from build123d import *

# Parameters (mm, degrees)
BOSS_EXTRUDE1_DEPTH     = 25.4
SKETCH2_W               = 12.7
SKETCH2_H               = 12.7
CUT_EXTRUDE1_DEPTH      = 12.7
MIRROR2_COPY_1_SKETCH_W = 12.7
MIRROR2_COPY_1_SKETCH_H = 12.7
MIRROR2_COPY_1_DEPTH    = 12.7
SKETCH3_R               = 3.175
CUT_EXTRUDE2_DEPTH      = 51.252303648


with BuildPart() as part:
    # Sketch1 → Boss-Extrude1 (new body)
    with BuildSketch(Plane.XY):
        Polygon((-30.660512242, 12.7), (-30.660512242, -12.7), (-12.7, -30.660512242), (12.7, -30.660512242), (30.660512242, -12.7), (30.660512242, 12.7), (12.7, 30.660512242), (-12.7, 30.660512242), align=None)
    extrude(amount=BOSS_EXTRUDE1_DEPTH)

    # Sketch2 → Cut-Extrude1 (cut)
    with BuildSketch(Plane(origin=(21.680256121, 21.680256121, 0), x_dir=(0, 0, -1), z_dir=(0.7071067811865479, 0.7071067811865472, 0))):
        with Locations((-12.7, 0)):
            Rectangle(SKETCH2_W, SKETCH2_H)
    cut_extrude1 = extrude(amount=-CUT_EXTRUDE1_DEPTH, mode=Mode.SUBTRACT)

    # Mirror1: Cut-Extrude1 across plane
    add(cut_extrude1.mirror(Plane(origin=(0, 0, 0), x_dir=(0, 0, 1), z_dir=(1, 0, 0))), mode=Mode.SUBTRACT)

    # Mirror2: Cut-Extrude1 across plane
    add(cut_extrude1.mirror(Plane.ZX), mode=Mode.SUBTRACT)

    # Mirror2 copy 1 sketch → Mirror2 copy 1 (cut)
    with BuildSketch(Plane(origin=(-21.680256121, -21.680256121, 0), x_dir=(0, 0, -1), z_dir=(-0.7071067811865472, -0.7071067811865479, 0))):
        with Locations((-12.7, 0)):
            Rectangle(MIRROR2_COPY_1_SKETCH_W, MIRROR2_COPY_1_SKETCH_H)
    extrude(amount=-MIRROR2_COPY_1_DEPTH, mode=Mode.SUBTRACT)

    # Sketch3 → Cut-Extrude2 (cut, through all)
    with BuildSketch(Plane.XY.offset(25.4)):
        with Locations((-17.190128061, 17.190128061)):
            Circle(SKETCH3_R)
        with Locations(Location((-17.190128061, -17.190128061, 0), (0, 0, 180))):
            Circle(SKETCH3_R)
        with Locations((17.190128061, -17.190128061)):
            Circle(SKETCH3_R)
        with Locations(Location((17.190128061, 17.190128061, 0), (0, 0, 180))):
            Circle(SKETCH3_R)
    extrude(amount=-CUT_EXTRUDE2_DEPTH, mode=Mode.SUBTRACT)


solid = part.part
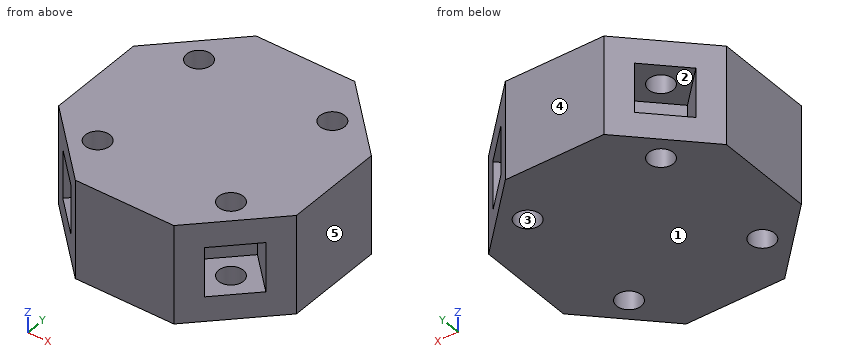
The listing builds one solid part. Answer for the finished solid, in the listing's coordinates (mm). Face numbers are marked on the shaded views. A direction names the side the tool comes from. Coordinates: 2 decimals unless noted, no trailing zeros. Loops run counter-clockwise (first coordinate to the right, second up) from the corner with the lowest first, then second, coordinate; pieces in that order, holes last.
1) Determine the mould class of the marked faces 3, 4 and 5 for opening direction X: pulls with the +X half, pulls with the -X half, needs draft (parallel to the pull), parting line crosses it, or undercut.
2) Find section D-D on x = 10. Write down the section's boundary in (y, z).
3) Find the intervals of material crossed by L1, parallel to Y at x = -17, z = 11; L2, parallel to Y at x = 9, z = 11; L3, parallel to X at y = -15.5, z = 1.25, in increasing order.
4) A tool of negligible diameter and unlimited length cuts with its end or side. For the marked faces 1 and 2, from which of +Z, -Z, +X, -X, +Y, -Y can it reach the whole face along a straight path? Write none if from no direction.
5) Find section B-B on x = -16. Write down the section's boundary in (y, z), then the cut area to 3 significant figures.
6) Flat-ended cylindrical pins translate along their axes: pin 1 Ø8 at (x, z) = (-24, 20.5) entering from +Y; pin 2 Ø9 at (x, y) = (15.5, -16.5) entering from -Z; pin 3 Ø4 at (x, z) = (-24, 17.5) entering from -Y; pin 4 Ø1 at (y, z) = (-21.5, 21.5) entering from +X. Find the tip coordinate at first contact, or state that the pin passes through.
7) Find section C-C on z = 13. Write down the section's boundary in (x, y), then the cut area to 3 significant figures.
8) Find section A-A on z = 22.25. Write down the section's boundary in (x, y) (3 decimals).
Values:
1. face 3: undercut
1. face 4: needs draft
1. face 5: pulls with the +X half
2. outline: (-30.66, 0) - (30.66, 0) - (30.66, 25.4) - (-30.66, 25.4) - close; hole (-18.98, 6.35) - (-15.4, 6.35) - (-15.4, 19.05) - (-18.98, 19.05) - close; hole (15.4, 6.35) - (18.98, 6.35) - (18.98, 19.05) - (15.4, 19.05) - close
3. L1: y = -26.36 to -25.98, -8.4 to 8.4, 25.98 to 26.36
3. L2: y = -30.66 to -17.98, -16.4 to 16.4, 17.98 to 30.66
3. L3: x = -27.86 to -19.88, -14.5 to 14.5, 19.88 to 27.86
4. face 1: -Z, +X, -X, +Y, -Y
4. face 2: none
5. outline: (-27.36, 0) - (-20.13, 0) - (-20.13, 6.35) - (-24.98, 6.35) - (-24.98, 19.05) - (-20.13, 19.05) - (-20.13, 25.4) - (-27.36, 25.4) - close; (-14.25, 0) - (14.25, 0) - (14.25, 6.35) - (9.4, 6.35) - (9.4, 19.05) - (14.25, 19.05) - (14.25, 25.4) - (-14.25, 25.4) - (-14.25, 19.05) - (-9.4, 19.05) - (-9.4, 6.35) - (-14.25, 6.35) - close; (20.13, 0) - (27.36, 0) - (27.36, 25.4) - (20.13, 25.4) - (20.13, 19.05) - (24.98, 19.05) - (24.98, 6.35) - (20.13, 6.35) - close
5. area: 845 mm2
6. pin 1: stops at y = 23.36
6. pin 2: stops at z = 0
6. pin 3: stops at y = -20.62
6. pin 4: stops at x = 22.36
7. outline: (-30.66, -12.7) - (-26.17, -17.19) - (-17.19, -8.21) - (-8.21, -17.19) - (-17.19, -26.17) - (-12.7, -30.66) - (12.7, -30.66) - (17.19, -26.17) - (8.21, -17.19) - (17.19, -8.21) - (26.17, -17.19) - (30.66, -12.7) - (30.66, 12.7) - (26.17, 17.19) - (17.19, 8.21) - (8.21, 17.19) - (17.19, 26.17) - (12.7, 30.66) - (-12.7, 30.66) - (-17.19, 26.17) - (-8.21, 17.19) - (-17.19, 8.21) - (-26.17, 17.19) - (-30.66, 12.7) - close
7. area: 2,470 mm2
8. outline: (-30.661, -12.7) - (-12.7, -30.661) - (12.7, -30.661) - (30.661, -12.7) - (30.661, 12.7) - (12.7, 30.661) - (-12.7, 30.661) - (-30.661, 12.7) - close; hole circle Ø6.35 at (-17.19, -17.19); hole circle Ø6.35 at (-17.19, 17.19); hole circle Ø6.35 at (17.19, -17.19); hole circle Ø6.35 at (17.19, 17.19)
